Can you work these out from the model? Positions are in its coordinate system, mm. A direction names the side the tool comes from. Round coordinates to 2 decimals unless told otherwise and drop trailing zeros. Order: outer loops, then holes, each group sorted by start corner. A loop starts at its lowest first (then second) coordinate and runs counter-clockwise, first axis right, second up. Notation, with made-up numbers: M -30,4.25 L 18,4.25 A35 cw 18,37.25 Z; hole C -31,22.5 d8. An arc over 180 degrees is marked long. One line per question, with ' | ' between items.
```python
from build123d import *

# Parameters (mm, degrees)
F0_W      = 8
F0_H      = 7.6
F1_DEPTH  = 38
F2_R      = 3
F3_R      = 3
F4_T      = -1.5
F5_W      = 8
F5_H      = 4.3
F6_DEPTH  = 7.6
F8_DEPTH  = 8.001
F9_W      = 5
F9_H      = 1.5
F10_DEPTH = 2.5
F12_DEPTH = 25
F14_W     = 1.3
F14_H     = 0.8
F16_R     = 0.5


with BuildPart() as f1:
    # F0 (on Front) → F1 (new body)
    with BuildSketch(Plane.XZ):
        with Locations((0, 3.8)):
            Rectangle(F0_W, F0_H)
    extrude(amount=-F1_DEPTH)

    # F2
    f2_edges = [f1.edges().sort_by_distance(p)[0] for p in [
        (4, 19, 7.6),
        (-4, 19, 7.6),
    ]]
    fillet(f2_edges, radius=F2_R)

    # F3
    f3_edges = [f1.edges().sort_by_distance(p)[0] for p in [
        (4, 38, 2.3),
    ]]
    fillet(f3_edges, radius=F3_R)

    # F4
    f4_openings = [f1.faces().sort_by_distance(p)[0] for p in [
        (0, 0, 3.587656),
    ]]
    offset(amount=F4_T, openings=f4_openings)

    # F5 (on face) → F6 (join)
    with BuildSketch(Plane.XZ):
        with Locations((0, 2.15)):
            Rectangle(F5_W, F5_H)
    extrude(amount=-F6_DEPTH)

    # F7 (on face) → F8 (cut, through all)
    with BuildSketch(Plane.YZ.offset(4)):
        Polygon((7.6, 7.6), (7.6, 4.3), (12.9, 7.6), align=None)
    extrude(amount=-F8_DEPTH, mode=Mode.SUBTRACT)

    # F9 (on face) → F10 (cut)
    with BuildSketch(Plane.XZ):
        with Locations((0, 3.55)):
            Rectangle(F9_W, F9_H)
    extrude(amount=-F10_DEPTH, mode=Mode.SUBTRACT)

    # F11 (on face) → F12 (cut)
    with BuildSketch(Plane.YZ.offset(4)):
        Polygon((8, 0), (0, 1.8), (0, 0), align=None)
    extrude(amount=-F12_DEPTH, mode=Mode.SUBTRACT)

    # F14 (on Right) → F15 (revolve)
    with BuildSketch(Plane.YZ):
        with Locations((40.15, 0.4)):
            Rectangle(F14_W, F14_H)
    revolve(axis=Axis((0, 38, 2.3), (0, 0, 1)))

    # F16
    f16_edges = [f1.edges().sort_by_distance(p)[0] for p in [
        (2.150942, 37.770439, 0.8),
        (-2.150942, 37.770439, 0.8),
        (2.743679, 37.441226, 0.4),
        (-2.743679, 37.441226, 0.4),
    ]]
    fillet(f16_edges, radius=F16_R)


solid = f1.part
```
(1) If we section it at B-B on y = 29: Please give me the cut outline in (x, z).
Final values:
outline: M -4,0 L 4,0 L 4,4.6 A3 ccw 1,7.6 L -1,7.6 A3 ccw -4,4.6 Z; hole M -2.5,1.5 L 2.5,1.5 L 2.5,4.6 A1.5 ccw 1,6.1 L -1,6.1 A1.5 ccw -2.5,4.6 Z
(2) If we section it at A-A on x = 0: Please give me the cut outline in (y, z), plus the area to 3 significant figures.
Final values:
outline: M 0,1.8 L 8,0 L 38,0 L 38,4.6 A3 ccw 35,7.6 L 12.9,7.6 L 10.49,6.1 L 35,6.1 A1.5 cw 36.5,4.6 L 36.5,1.5 L 7.6,1.5 L 7.6,4.3 L 2.5,4.3 L 2.5,2.8 L 0,2.8 Z; M 0,6.1 L 7.6,6.1 L 7.6,7.6 L 0,7.6 Z; M 39.5,0 L 40.8,0 L 40.8,0.8 L 39.5,0.8 Z | area: 125 mm^2
(3) If we section it at D-D on y = 36: Please give me the cut outline in (x, z).
Final values:
outline: M -3.83,0 L 3.83,0 L 3.83,4.6 A2.83 ccw 1,7.43 L -1,7.43 A2.83 ccw -3.83,4.6 Z; hole M -2.12,1.5 L 2.12,1.5 L 2.12,4.6 A1.12 ccw 1,5.72 L -1,5.72 A1.12 ccw -2.12,4.6 Z
(4) Will these pins go through, and if not, where does the flat tip stop? pin 1 Ø1.6 at (x, z) = (0, 4) entering from -Y; pin 2 Ø1.5 at (x, y) = (-3, 4.5) entering from +Z; pin 3 Ø3 at (x, y) = (1.5, 40) entering from +Z.
Final values:
pin 1: y = 2.5 | pin 2: z = 7.33 | pin 3: z = 0.8
(5) If we section it at C-C on z = 3.75: Please give me the cut outline in (x, y).
Final values:
outline: M -4,0 L -2.5,0 L -2.5,2.5 L 2.5,2.5 L 2.5,0 L 4,0 L 4,35 A3 ccw 1,38 L -1,38 A3 ccw -4,35 Z; hole M -2.5,7.6 L 2.5,7.6 L 2.5,35 A1.5 ccw 1,36.5 L -1,36.5 A1.5 ccw -2.5,35 Z
(6) On a 3-axis mill with a long thin cutter (end or side, diameter ignored), from which of +Z, -Z, +X, -X, +Y, -Y can I reach the whole of each face in a straight line? I mean faces 4 (the flat face through (4, 17, 2)), 5 (the cylindrical face through (-2.07, 21.73, 5.65)), 6 (the flat face through (-2.5, 21, 3)). Say none if no direction works.
Final values:
face 4: +Z, -Z, +X, +Y, -Y | face 5: -Y | face 6: none
(7) Thinking about a two-plate mould opening in X: for faces 1 (the cylindrical face through (3.14, 3.85, 6.7)), 2 (the flat face through (0.056, 4.056, 0.887)), 3 (the flat face through (-2.5, 2, 4)), which applies, released by +X, released by -X, zero draft, split by the parting line, or undercut?
Final values:
face 1: released by +X | face 2: zero draft | face 3: undercut
(8) Please list where these lines run through material, in increasing order: probe 1 along Z at (x, y) = (-0.25, 25); probe 2 along Y at (x, z) = (0.5, 3); probe 3 along X at (y, z) = (19, 4). Write a range as [from, to].
Final values:
probe 1: [0, 1.5], [6.1, 7.6] | probe 2: [2.5, 7.6], [36.5, 38] | probe 3: [-4, -2.5], [2.5, 4]
